Read the model definition and answer for the solid it produces. Units are mm, in the model's axes. Give positions to 0.01 mm unless a question says otherwise; leave off trailing zeros. Order: outer loops, then holes, each group sorted by start corner. A loop starts at its lowest first (then second) coordinate and runs counter-clockwise, first axis right, second up. Notation, with made-up numbers: M 60,-6.5 L 109,-6.5 A10 cw 109,8.5 Z; hole C -40,13 d4. An arc over 180 degrees is marked long. One line per item, written item: value.
from build123d import *

# Parameters (mm, degrees)
F1_W     = 6
F1_H     = 3
F2_DEPTH = 3
F3_R     = 5


with BuildPart() as f2:
    # F1 (on Top) → F2 (new body)
    with BuildSketch(Plane.XY):
        Polygon((39.5, -49), (45.5, -49), (45.5, 49), (-45.5, 49), (-45.5, -49), (36.5, -49), (36.5, 0), (39.5, 0), align=None)
        with Locations((-8.5, -37.5)):
            Rectangle(F1_W, F1_H, mode=Mode.SUBTRACT)
        with Locations((-8.5, 37.5)):
            Rectangle(F1_W, F1_H, mode=Mode.SUBTRACT)
        with BuildLine():
            Line((45.5, 49), (45.5, -49))
            Line((45.5, -49), (48.5, -49))
            ThreePointArc((48.5, -49), (46.5, 0), (48.5, 49))
            Line((48.5, 49), (45.5, 49))
        make_face()
        with BuildLine():
            Line((36.5, -49.8917956467), (36.5, -49))
            Line((36.5, -49), (-45.5, -49))
            ThreePointArc((-45.5, -49), (-4.5165459251, -50.9672843243), (36.5, -49.8917956467))
        make_face()
        with BuildLine():
            Line((48.5, -49), (45.5, -49))
            Line((45.5, -49), (39.5, -49))
            Line((39.5, -49), (39.5, -49.6934413959))
            ThreePointArc((39.5, -49.6934413959), (44.0014142734, -49.3650761942), (48.5, -49))
        make_face()
        with BuildLine():
            Line((-45.5, 49), (45.5, 49))
            Line((45.5, 49), (48.5, 49))
            ThreePointArc((48.5, 49), (1.5, 51), (-45.5, 49))
        make_face()
        with BuildLine():
            Line((-45.5, -49), (-45.5, 49))
            ThreePointArc((-45.5, 49), (-47.5, 0), (-45.5, -49))
        make_face()
    extrude(amount=F2_DEPTH)

    # F3
    f3_edges = [f2.edges().sort_by_distance(p)[0] for p in [
        (-45.5, -49, 1.5),
        (-45.5, 49, 1.5),
        (48.5, -49, 1.5),
        (48.5, 49, 1.5),
    ]]
    fillet(f3_edges, radius=F3_R)


solid = f2.part
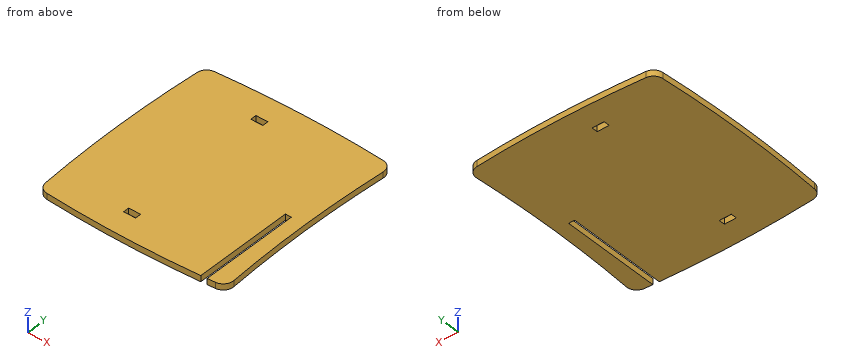
1) Each of these flat-tipped pins is pushed along its axis until it touches: pin 1 Ø1.5 at (x, z) = (-10, 1.5) entering from +Y; pin 2 Ø0.9 at (y, z) = (-37, 1.5) entering from +X; pin 3 Ø1.5 at (y, z) = (37.5, 2) entering from -X. Where does it stop, or does it pass through?
Reported:
pin 1: stops at y = 50.9
pin 2: stops at x = 47.67
pin 3: stops at x = -46.38
2) Find section A-A, the plane x = -8.5. Write down the section's boundary in (y, z).
Reported:
outline: M -50.91,0 L -39,0 L -39,3 L -50.91,3 Z; M -36,0 L 36,0 L 36,3 L -36,3 Z; M 39,0 L 50.91,0 L 50.91,3 L 39,3 Z
3) Find section C-C, the plane z = 1. Count the separate pieces of the cut face and the enclosed holes in it, plus the area to 3 significant figures.
Reported:
separate pieces: 1
enclosed holes: 2
area: 9,260 mm^2
4) Consider probe 1 along Y at (x, z) = (-11, 2.05); probe 2 along X at (y, z) = (-37, 2.25); probe 3 along X at (y, z) = (-45.5, 1). Determine where each line is inside the solid, lowest interval first.
Reported:
probe 1: y = -50.86 to -39, -36 to 36, 39 to 50.86
probe 2: x = -46.36 to -11.5, -5.5 to 36.5, 39.5 to 47.64
probe 3: x = -45.72 to 36.5, 39.5 to 48.01
5) Find section B-B, the plane y = -9. Write down the section's boundary in (x, z), plus the area to 3 significant figures.
Reported:
outline: M -47.43,0 L 36.5,0 L 36.5,3 L -47.43,3 Z; M 39.5,0 L 46.57,0 L 46.57,3 L 39.5,3 Z
area: 273 mm^2
6) Find section D-D, the plane x = 41. Write down the section's boundary in (y, z), plus the area to 3 significant figures.
Reported:
outline: M -49.59,0 L 49.59,0 L 49.59,3 L -49.59,3 Z
area: 298 mm^2
